The listing builds one solid part. Answer for the finished solid, in the listing's coordinates (mm). Face numbers are marked on the shaded views. Round coordinates to 2 decimals unless told otherwise and drop trailing zeros. Write each loop counter-clockwise with the first axis right and the second up, starting at its lowest first coordinate (ties: lowest second). Pieces come first, ordered by that corner, then holes. Notation, with made-up numbers: (-7.75, 68.25) - (50.25, 68.25) arc R9 ccw to (50.25, 85.25) - close; hole circle Ø11 at (83, 45.25). An arc over 180 degrees is marked (long way). Use a Markdown table: item, result. Add a question column.
1) A cutting plane is placed at D-D (z = 27.5). Give the vertices of the cut face in (x, y).
2) A cutting plane is placed at C-C (y = -7). Give the vertices of the cut face in (x, z), then the cut area to 3 significant figures.
3) Each of these flat-tipped pins is pushed along its axis until it touches: P1, Ø5, axis at y = 9, z = 47, coming from the -X side; P2, Ø1, axis at x = -5, z = 34.5, coming from the -Y side; P3, Ø6, axis at x = -5, z = 83, coming from the -Y side. Where does it stop, or does it pass through?
4) Find the intervals of material crossed by probe 1 along Z at (x, y) = (10.8, 0); probe 2 along X at (y, z) = (0, 33.5); probe 3 along X at (y, z) = (-8.25, 28.5), in increasing order. Write a range as from..to.
5) A cutting plane is placed at B-B (x = 0). Give the vertices of the cut face in (y, z), then the cut area to 3 significant figures.
6) A cutting plane is placed at A-A (y = 0). Give the vertices of the cut face in (x, z).
7) Determine the mould class of the marked faces 1 and 2 for opening direction Y: +Y half, -Y half, draft (parallel to the pull), parting line (faces both ways), or undercut.
```python
from build123d import *

# Parameters (mm, degrees)
F0_R     = 12.5
F1_DEPTH = 100
F2_T     = -2
F5_D     = 8


with BuildPart() as f1:
    # F0 (on Top) → F1 (new body)
    with BuildSketch(Plane.XY):
        Circle(F0_R)
    extrude(amount=F1_DEPTH)

    # F2
    f2_openings = [f1.faces().sort_by_distance(p)[0] for p in [
        (0, 0, 100),
        (0, 0, 0),
    ]]
    offset(amount=F2_T, openings=f2_openings)

    # F5 (through all)
    with Locations(Plane(origin=(-30, 0, 0), x_dir=(0, 1, 0), z_dir=(-1, 0, 0))):
        with Locations((0, -10)):
            Hole(F5_D / 2)


solid = f1.part
```
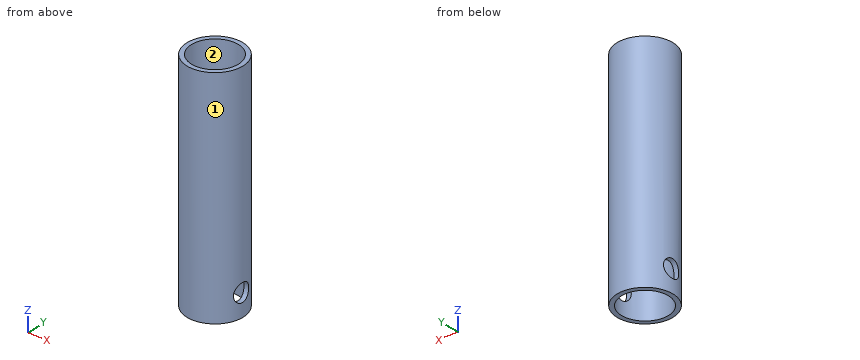
Entries:
| question | item | result |
|---|---|---|
| 1 | outline | circle Ø25 at (0, 0); hole circle Ø21 at (0, 0) |
| 2 | outline | (-10.36, 0) - (-7.83, 0) - (-7.83, 100) - (-10.36, 100) - close; (7.83, 0) - (10.36, 0) - (10.36, 100) - (7.83, 100) - close |
| 2 | area | 506 mm² |
| 3 | P1 | stops at x = -10.68 |
| 3 | P2 | stops at y = -11.66 |
| 3 | P3 | stops at y = -12.34 |
| 4 | probe 1 | z = 0..6, 14..100 |
| 4 | probe 2 | x = -12.5..-10.5, 10.5..12.5 |
| 4 | probe 3 | x = -9.39..-6.5, 6.5..9.39 |
| 5 | outline | (-12.5, 0) - (-10.5, 0) - (-10.5, 100) - (-12.5, 100) - close; (10.5, 0) - (12.5, 0) - (12.5, 100) - (10.5, 100) - close |
| 5 | area | 400 mm² |
| 6 | outline | (-12.5, 0) - (-10.5, 0) - (-10.5, 6) - (-12.5, 6) - close; (-12.5, 14) - (-10.5, 14) - (-10.5, 100) - (-12.5, 100) - close; (10.5, 0) - (12.5, 0) - (12.5, 6) - (10.5, 6) - close; (10.5, 14) - (12.5, 14) - (12.5, 100) - (10.5, 100) - close |
| 7 | face 1 | parting line |
| 7 | face 2 | undercut |
